Autodesk Inventor part; units mm, degrees
ref_plane "YZ Plane" through (0, 0, 0) normal (1, 0, 0) x (0, 1, 0)
ref_plane "XZ Plane" through (0, 0, 0) normal (0, 1, 0) x (-1, 0, 0)
ref_plane "XY Plane" through (0, 0, 0) normal (0, 0, 1) x (1, 0, 0)
sketch "Sketch1" plane through (0, 0, 0) normal (0, 1, 0) x (-1, 0, 0)
  line L0 (7.25, 7.25) -> (-7.25, 7.25)
  line L1 (-7.25, 7.25) -> (-7.25, -7.25)
  line L2 (-7.25, -7.25) -> (7.25, -7.25)
  line L3 (7.25, -7.25) -> (7.25, 7.25)
  circle A0 centre (6, 0) radius 0.8
  circle A1 centre (-6, 0) radius 0.8
  circle A2 centre (6, 0) radius 1.5
  circle A3 centre (-6, 0) radius 1.5
  point P0 (0, 0)
  point P1 (7.25, 0)
  point P2 (0, -7.25)
  dimension "d0" = 14.5
  dimension "d1" = 1.6
  dimension "d3" = 3
  dimension "d4" = 6
  dimension "d5" = 6
extrude "Extrusion1" add sketch "Sketch1" along normal blind 2 contours L3 A2 L2 L1 A3 L0
extrude "Extrusion2" add sketch "Sketch1" along normal blind 0.5 contours A2 L3 | L3 A2 | A3 L1 | L1 A3
properties part number "temp apd reinforcement"
Build history of the part. All positions in model axes, mm. A direction names the side the tool comes from. Round coordinates to 2 decimals unless told otherwise and drop trailing zeros. Loops run counter-clockwise (first coordinate to the right, second up) from the corner with the lowest first, then second, coordinate; pieces in that order, holes last.
Item 1: Two-plate mould, pull along Z, no slides. Class faces 6 (the face through (-7, 0.5, 0)), 7 (the face through (-5.2, 0.2, 0)), 8 (the face through (-7.25, 1, -4)), 9 (the face through (0, 1, -7.25)): released by +Z, released by -Z, zero draft, split by the parting line, or undercut.
Item 2: Saw through at B-B (x = -6). List the corners of the cut face in (y, z).
Item 3: Which spindle directions (+Z, -Z, +X, -X, +Y, -Y) get a long thin tool onto all of the face, cutting with end or side? Do faces 1 (the face through (-7.25, 1, 4)), 2 (the face through (6.8, 0.2, 0)), 3 (the face through (7.25, 1, 4)), 4 (the face through (7.25, 1, -4)), 5 (the face through (4.5, 1.24, 0.05)). Say none if no direction does.
Item 4: Saw through at A-A (z = 0). List the corners of the cut face in (x, y).
Item 5: Drill centre lines: line 1 along Z through (x, y) = (6, 0.2); line 2 along X through (y, z) = (1.3, 0); line 3 along X through (y, z) = (1.15, 3). Where is each one in solid material? Low to high.
Item 6: Saw through at D-D (x = 6.5). List the corners of the cut face in (y, z).
Item 7: Pin check, flat tips, straight feed: P1, Ø1, axis at y = 1, z = -5, coming from the -X side; P2, Ø2, axis at x = -6, z = 0, coming from the +Y side; P3, Ø0.6, axis at y = 0.5, z = -3.5, coming from the +X side. Stop position of each tip, or through.
Item 8: Saw through at C-C (y = 1.55). List the corners of the cut face in (x, z), then the cut area to 3 significant figures.
Worked answers:
1. face 6: undercut
1. face 7: undercut
1. face 8: zero draft
1. face 9: released by -Z
2. outline: (0, -7.25) - (2, -7.25) - (2, -1.5) - (0.5, -1.5) - (0.5, -0.8) - (0, -0.8) - close; (0, 0.8) - (0.5, 0.8) - (0.5, 1.5) - (2, 1.5) - (2, 7.25) - (0, 7.25) - close
3. face 1: +Z, -X, +Y, -Y
3. face 2: +Y, -Y
3. face 3: +Z, +X, +Y, -Y
3. face 4: -Z, +X, +Y, -Y
3. face 5: +Y
4. outline: (-7.5, 0) - (-6.8, 0) - (-6.8, 0.5) - (-7.5, 0.5) - close; (-5.2, 0) - (5.2, 0) - (5.2, 0.5) - (4.5, 0.5) - (4.5, 2) - (-4.5, 2) - (-4.5, 0.5) - (-5.2, 0.5) - close; (6.8, 0) - (7.5, 0) - (7.5, 0.5) - (6.8, 0.5) - close
5. line 1: z = -7.25 to -0.8, 0.8 to 7.25
5. line 2: x = -4.5 to 4.5
5. line 3: x = -7.25 to 7.25
6. outline: (0, -7.25) - (2, -7.25) - (2, -1.41) - (0.5, -1.41) - (0.5, -0.62) - (0, -0.62) - close; (0, 0.62) - (0.5, 0.62) - (0.5, 1.41) - (2, 1.41) - (2, 7.25) - (0, 7.25) - close
7. P1: stops at x = -7.25
7. P2: stops at y = 0.5
7. P3: stops at x = 7.25
8. outline: (-7.25, -7.25) - (7.25, -7.25) - (7.25, -0.83) arc R1.5 cw (long way) to (7.25, 0.83) - (7.25, 7.25) - (-7.25, 7.25) - (-7.25, 0.83) arc R1.5 cw (long way) to (-7.25, -0.83) - close
8. area: 197 mm2
